The model under review builds one solid part; all positions refer to its coordinate system, in mm. A direction names the side the tool comes from. Coordinates: 2 decimals unless noted, no trailing zeros. Order: outer loops, then holes, each group sorted by start corner. A loop starts at its lowest first (then second) coordinate and runs counter-clockwise, first axis right, second up. Notation, with made-up numbers: M -9.5,-40 L 46.5,-40 A13 ccw 46.5,-35 Z; hole C 24.5,54.25 d4. An arc over 180 degrees is marked long. One line per item, written item: value.
```python
from build123d import *

# Parameters (mm, degrees)
BOSS_EXTRUDE1_DEPTH = 6


with BuildPart() as part:
    # Sketch1 → Base-Revolve (revolve)
    with BuildSketch(Plane(origin=(0, 0, 0), x_dir=(1, 0, 0), z_dir=(0, 1, 0))):
        Polygon((0, 0), (0, -40), (2.75, -40), (2.75, -36), (4, -36), (4, 0), align=None)
    revolve(axis=Axis((0, 0, -1.187299328), (0, 0, 1)))

    # Sketch2 → Boss-Extrude1 (add)
    with BuildSketch(Plane(origin=(0, 0, 0), x_dir=(-1, 0, 0), z_dir=(0, 0, -1))):
        Polygon((5, -2.886751346), (5, 2.886751346), (0, 5.773502692), (-5, 2.886751346), (-5, -2.886751346), (0, -5.773502692), align=None)
    extrude(amount=BOSS_EXTRUDE1_DEPTH)


solid = part.part
```
(1) We need section A-A, the plane y = 0. State the section outline as (x, z) points, plus the area to 3 significant figures.
Geometry results:
outline: M -5,-6 L 5,-6 L 5,0 L 4,0 L 4,36 L 2.75,36 L 2.75,40 L -2.75,40 L -2.75,36 L -4,36 L -4,0 L -5,0 Z
area: 370 mm2
(2) Tool access review of faces 1 (the flat face through (0, 0, 40)), 2 (the cylindrical face through (-0.596, -2.685, 37.972)): name each direction out of +Z, -Z, +X, -X, +Y, -Y from which nothing blocks a thin tool from reaching the whole face with its end or side.
Geometry results:
face 1: +Z, +X, -X, +Y, -Y
face 2: +Z
(3) We need section B-B, the plane z = 33. State the section outline as (x, y) points.
Geometry results:
outline: C 0,0 d8
(4) For L1, parallel to Z at x = 3.5, y = -1.75; L2, parallel to Z at x = 4.25, y = 0.5; L3, parallel to Y at x = 0, z = 1.5, list the stretches that pass through material, from the lowest coordinate up.
Geometry results:
L1: z = -6 to 36
L2: z = -6 to 0
L3: y = -4 to 4
(5) We need section D-D, the plane y = -1.75. State the section outline as (x, z) points, plus the area to 3 significant figures.
Geometry results:
outline: M -5,-6 L 5,-6 L 5,0 L 3.6,0 L 3.6,36 L 2.12,36 L 2.12,40 L -2.12,40 L -2.12,36 L -3.6,36 L -3.6,0 L -5,0 Z
area: 336 mm2
(6) We need section C-C, the plane x = 3.5. State the section outline as (y, z) points.
Geometry results:
outline: M -3.75,-6 L 3.75,-6 L 3.75,0 L 1.94,0 L 1.94,36 L -1.94,36 L -1.94,0 L -3.75,0 Z
(7) Insertion check: pin 1 Ø6 at (x, z) = (-2.5, 27) entering from +Y; pin 2 Ø4 at (x, y) = (3.5, 4) entering from +Z; pin 3 Ø1.5 at (y, z) = (2.5, 4.5) entering from +X. Each pin has a flat end and moves straight along its axis. Give the tip position at first contact, or say it passes through.
Geometry results:
pin 1: stops at y = 4
pin 2: stops at z = 36
pin 3: stops at x = 3.6
